from build123d import *

# Parameters (mm, degrees)
SKETCH1_W                = 22.5
SKETCH1_H                = 7
BOSS_EXTRUDE1_DEPTH      = 1.5
SKETCH2_R                = 1.475
BOSS_EXTRUDE2_DEPTH      = 11.5
BOSS_EXTRUDE4_DEPTH      = 6
BOSS_EXTRUDE4_DEPTH_BACK = 1.5
SKETCH4_W                = 22.5
SKETCH4_H                = 2.5
SKETCH4_H_2              = 7
SKETCH8_W                = 22.5
SKETCH8_H                = 9.5
BOSS_EXTRUDE7_DEPTH      = 2.61
BOSS_EXTRUDE8_DEPTH      = 7.76
BOSS_EXTRUDE8_DEPTH_BACK = 1.5
SKETCH9_R                = 2.4
SKETCH15_W               = 9.5
SKETCH15_H               = 3
BOSS_EXTRUDE11_DEPTH     = 4.5
SKETCH16_W               = 1.5
SKETCH16_H               = 9.5
CUT_EXTRUDE3_DEPTH       = 1.5
FILLET1_SIZE             = 4.5
FILLET1_SIZE_2           = 1.5
FILLET2_R                = 1.5
FILLET3_R                = 1.5
FILLET4_R                = 2
FILLET5_R                = 0.75
FILLET9_SIZE             = 5
FILLET9_SIZE_2           = 2.5


with BuildPart() as part:
    # Sketch1 → Boss-Extrude1 (new body)
    with BuildSketch(Plane(origin=(0, 0, 0), x_dir=(1, 0, 0), z_dir=(0, 1, 0))):
        with Locations((-28.93578967, -21.079480712)):
            Rectangle(SKETCH1_W, SKETCH1_H)
    extrude(amount=BOSS_EXTRUDE1_DEPTH)

    # Sketch2 → Boss-Extrude2 (add)
    with BuildSketch(Plane(origin=(0, 1.5, 0), x_dir=(1, 0, 0), z_dir=(0, 1, 0))):
        with Locations(Location((-37.53578967, -19.579480712, 0), (0, 0, 90))):
            Circle(SKETCH2_R)
        with Locations(Location((-20.33578967, -19.579480712, 0), (0, 0, 90))):
            Circle(SKETCH2_R)
    extrude(amount=BOSS_EXTRUDE2_DEPTH)

    # Sketch4 → Boss-Extrude4 (add, two sides: drawn at the far end of the back side and taken through both)
    with BuildSketch(Plane(origin=(0, 0, 0), x_dir=(-1, 0, 0), z_dir=(0, -1, 0)).offset(-BOSS_EXTRUDE4_DEPTH_BACK)):
        with Locations((28.93578967, -25.829480712)):
            Rectangle(SKETCH4_W, SKETCH4_H)
        with Locations((28.93578967, -21.079480712)):
            Rectangle(SKETCH4_W, SKETCH4_H_2)
    extrude(amount=BOSS_EXTRUDE4_DEPTH + BOSS_EXTRUDE4_DEPTH_BACK)

    # Sketch8 → Boss-Extrude7 (add)
    with BuildSketch(Plane(origin=(0, 1.5, 0), x_dir=(1, 0, 0), z_dir=(0, 1, 0))):
        with Locations((-28.93578967, -22.329480712)):
            Rectangle(SKETCH8_W, SKETCH8_H)
    extrude(amount=BOSS_EXTRUDE7_DEPTH)

    # Sketch9 → Boss-Extrude8 (add, two sides: drawn at the far end of the back side and taken through both)
    with BuildSketch(Plane(origin=(0, -6, 0), x_dir=(-1, 0, 0), z_dir=(0, -1, 0)).offset(-BOSS_EXTRUDE8_DEPTH_BACK)):
        with Locations(Location((28.81078967, -25.489480712, 0), (0, 0, 90))):
            Circle(SKETCH9_R)
        with Locations(Location((28.81078967, -17.519480712, 0), (0, 0, 90))):
            Circle(SKETCH9_R)
    extrude(amount=BOSS_EXTRUDE8_DEPTH + BOSS_EXTRUDE8_DEPTH_BACK)

    # Sketch15 → Boss-Extrude11 (add)
    with BuildSketch(Plane.ZY.offset(40.18578967)):
        with Locations((22.329480712, -2.09)):
            Rectangle(SKETCH15_W, SKETCH15_H)
    extrude(amount=BOSS_EXTRUDE11_DEPTH)

    # Sketch16 → Cut-Extrude3 (cut)
    with BuildSketch(Plane(origin=(0, -0.59, 0), x_dir=(1, 0, 0), z_dir=(0, 1, 0))):
        with Locations((-42.43578967, -22.329480712)):
            Rectangle(SKETCH16_W, SKETCH16_H)
    extrude(amount=-CUT_EXTRUDE3_DEPTH, mode=Mode.SUBTRACT)

    # Fillet1
    # an asymmetric fillet: 4.5, 1.5 mm, written as the material it adds along each edge
    with BuildSketch(Plane(origin=(-40.18578967, -0.59, 27.079480712), x_dir=(0, 1, 0), z_dir=(0, 0, -1))) as fillet1_piece_1:
        with BuildLine():
            Bezier((FILLET1_SIZE, 0), (0, 0), (0, -FILLET1_SIZE_2), weights=[1, 0.707106781, 1])
            Line((0, -FILLET1_SIZE_2), (0, 0))
            Line((0, 0), (FILLET1_SIZE, 0))
        make_face()
    extrude(amount=9.5)

    # Fillet2
    fillet2_edges = [part.edges().sort_by_distance(p)[0] for p in [
        (-44.68578967, -3.59, 22.329480712),
    ]]
    fillet(fillet2_edges, radius=FILLET2_R)

    # Fillet3
    fillet3_edges = [part.edges().sort_by_distance(p)[0] for p in [
        (-40.18578967, -3.59, 22.329480712),
    ]]
    fillet(fillet3_edges, radius=FILLET3_R)

    # Fillet4
    fillet4_edges = [part.edges().sort_by_distance(p)[0] for p in [
        (-28.81078967, -4.5, 17.579480712),
    ]]
    fillet(fillet4_edges, radius=FILLET4_R)

    # Fillet5
    fillet5_edges = [part.edges().sort_by_distance(p)[0] for p in [
        (-28.81078967, -4.5, 27.079480712),
    ]]
    fillet(fillet5_edges, radius=FILLET5_R)

    # Fillet9
    # an asymmetric fillet: 5, 2.5 mm, written as the material it takes off along each edge
    with BuildSketch(Plane(origin=(-17.68578967, 16.61, 17.579480712), x_dir=(-1, 0, 0), z_dir=(0, -1, 0))) as fillet9_piece_1:
        with BuildLine():
            Bezier((FILLET9_SIZE, 0), (0, 0), (0, -FILLET9_SIZE_2), weights=[1, 0.707106781, 1])
            Line((0, -FILLET9_SIZE_2), (0, 0))
            Line((0, 0), (FILLET9_SIZE, 0))
        make_face()
    extrude(amount=35.11, mode=Mode.SUBTRACT)


solid = part.part
Can you work these out from the model? Positions are in its coordinate system, mm. A direction names the side the tool comes from. Coordinates: 2 decimals unless noted, no trailing zeros. Write each loop counter-clockwise with the first axis right and the second up, starting at its lowest first coordinate (ties: lowest second). Pieces come first, ordered by that corner, then holes. Notation, with made-up numbers: (-11.75, -39) -> (-5.75, -39) arc R10 ccw to (-5.75, -22) -> close; hole circle Ø7 at (-2, -32.75). An arc over 180 degrees is marked (long way). Write each question's results on one line, items separated by ' | '. Start each with the question number.
Q1. I'm going to push flat-ended pins straight in: pin 1 (2 mm diameter, centred on x = -25.5, z = 21, fed in from +Y); pin 2 (0.7 mm diameter, centred on y = -5.5, z = 24, fed in from -X); pin 3 (5 mm diameter, centred on x = -29, y = 0.5, fed in from -Z). Where does each tip first touch, or does it pass through?
Q2. Imagine slicing it at C-C (z = 17.25). Write out the boundary of the cut face in (x, y).
Q3. Imagine slicing it at A-A (y = 5.5). Write out the boundary of the cut face in (x, z) (3 decimals).
Q4. We'd pull the mould along X, two halves only. Please class faces 6 (the face through (-44, -0.59, 22)), 7 (the face through (-40.637, -4.018, 22.396)), 8 (the face through (-36.64, 8.49, 20.75)): +X half, -X half, draft (parallel to the pull), parting line (faces both ways), or undercut.
Q5. Imagine slicing it at B-B (x = -39.5). Write out the boundary of the cut face in (y, z), then the cut area to 3 significant figures.
Q6. If I drill on probe 1 along X at (y, z) = (-1, 26.5); probe 2 along Z at (x, y) = (-31, -6.5); probe 3 along Y at (x, z) = (-19.5, 19), over which ranges is the centre line in solid material (lowest first)?
Q7. Imagine slicing it at D-D (y = -11.75). Write out the boundary of the cut face in (x, z).
Q8. On a 3-axis mill with a long thin cutter (end or side, diameter ignored), from which of +Z, -Z, +X, -X, +Y, -Y can I reach the whole of each face in a straight line? I mean faces 1 (the face through (-44.686, -1, 22)), 2 (the face through (-28.705, -9.797, 27.887)), 3 (the face through (-42, -3.59, 22)), 4 (the face through (-29, -13.76, 26)), 5 (the face through (-42, -2.09, 22)). Say none if no direction works.
Taken from the geometry:
1) pin 1: stops at y = 4.11 | pin 2: stops at x = -40.19 | pin 3: stops at z = 17.58
2) outline: (-31.2, -13.76) -> (-26.43, -13.76) -> (-26.43, -3.6) -> (-31.2, -3.6) -> close
3) outline: circle Ø2.95 at (-37.536, 19.579); circle Ø2.95 at (-20.336, 19.579)
4) face 6: draft | face 7: -X half | face 8: undercut
5) outline: (-6, 17.58) -> (4.11, 17.58) -> (4.11, 27.08) -> (-6, 27.08) -> close | area: 96.0 mm^2
6) probe 1: x = -44.69 to -43.19, -41.69 to -17.69 | probe 2: z = 16.54 to 18.5, 24.51 to 26.47 | probe 3: y = -6 to 13
7) outline: circle Ø4.8 at (-28.81, 17.52); circle Ø4.8 at (-28.81, 25.49)
8) face 1: +Z, -Z, -X, +Y, -Y | face 2: -Y | face 3: +Z, -Z, -X, -Y | face 4: +Z, -Z, +X, -X, -Y | face 5: +Z, -Z, +Y
